```python
from build123d import *

# Parameters (mm, degrees)
SKETCH1_W           = 16
SKETCH1_H           = 20
BOSS_EXTRUDE1_DEPTH = 1.5
SKETCH2_R           = 1.5
CUT_EXTRUDE1_DEPTH  = 3
FILLET1_R           = 2


with BuildPart() as part:
    # Sketch1 → Boss-Extrude1 (new, symmetric)
    with BuildSketch(Plane(origin=(0, 0, 0), x_dir=(1, 0, 0), z_dir=(0, 1, 0))):
        Rectangle(SKETCH1_W, SKETCH1_H)
    extrude(amount=BOSS_EXTRUDE1_DEPTH, both=True)

    # Sketch2 → Cut-Extrude1 (cut)
    with BuildSketch(Plane(origin=(0, 1.5, 0), x_dir=(1, 0, 0), z_dir=(0, 1, 0))):
        with Locations(Location((-4, -4.5, 0), (0, 0, 270))):
            Circle(SKETCH2_R)
        with Locations(Location((-4, 4.5, 0), (0, 0, 270))):
            Circle(SKETCH2_R)
        with Locations(Location((4, 4.5, 0), (0, 0, 270))):
            Circle(SKETCH2_R)
        with Locations(Location((4, -4.5, 0), (0, 0, 270))):
            Circle(SKETCH2_R)
    extrude(amount=-CUT_EXTRUDE1_DEPTH, mode=Mode.SUBTRACT)

    # Fillet1
    fillet1_edges = [part.edges().sort_by_distance(p)[0] for p in [
        (8, 0, 10),
        (-8, 0, 10),
        (-8, 0, -10),
        (8, 0, -10),
    ]]
    fillet(fillet1_edges, radius=FILLET1_R)


solid = part.part
```
Input: part model. Units: mm. Frame: model coordinates. Give positions to 0.01 mm unless a question says otherwise; leave off trailing zeros. Loops run counter-clockwise (first coordinate to the right, second up) from the corner with the lowest first, then second, coordinate; pieces in that order, holes last.
1) Section query A-A on x = 4. Return the cut outline in (y, z), and give its area (3 significant figures).
A:
outline: (-1.5, -10) - (1.5, -10) - (1.5, -6) - (-1.5, -6) - close; (-1.5, -3) - (1.5, -3) - (1.5, 3) - (-1.5, 3) - close; (-1.5, 6) - (1.5, 6) - (1.5, 10) - (-1.5, 10) - close
area: 42.0 mm2
2) Line query: L1, parallel to X at y = 0, z = 4.5; L2, parallel to Z at x = -3.5, y = 0.6; L3, parallel to Z at x = -5, y = 0.05. Output: solid intervals per line, ascending.
A:
L1: x = -8 to -5.5, -2.5 to 2.5, 5.5 to 8
L2: z = -10 to -5.91, -3.09 to 3.09, 5.91 to 10
L3: z = -10 to -5.62, -3.38 to 3.38, 5.62 to 10
3) Section query B-B on z = 4.5. Return the cut outline in (x, y), and give its area (3 significant figures).
A:
outline: (-8, -1.5) - (-5.5, -1.5) - (-5.5, 1.5) - (-8, 1.5) - close; (-2.5, -1.5) - (2.5, -1.5) - (2.5, 1.5) - (-2.5, 1.5) - close; (5.5, -1.5) - (8, -1.5) - (8, 1.5) - (5.5, 1.5) - close
area: 30.0 mm2
4) Mould query, pull axis X, two halves, no side actions, for faces 1 (the cylindrical face through (4, 0, 6)), 2 (the cylindrical face through (-4, 0, 6)), 3 (the flat face through (-8, 0, 0)), 4 (the cylindrical face through (7.4, 0.02, 9.43)). Classes: released by +X, released by -X, zero draft, split by the parting line, or undercut.
A:
face 1: undercut
face 2: undercut
face 3: released by -X
face 4: released by +X
5) Section query C-C on y = -0.85. Return the cut outline in (x, z), and give its area (3 significant figures).
A:
outline: (-8, -8) arc R2 ccw to (-6, -10) - (6, -10) arc R2 ccw to (8, -8) - (8, 8) arc R2 ccw to (6, 10) - (-6, 10) arc R2 ccw to (-8, 8) - close; hole circle Ø3 at (-4, -4.5); hole circle Ø3 at (-4, 4.5); hole circle Ø3 at (4, -4.5); hole circle Ø3 at (4, 4.5)
area: 288 mm2
